from build123d import *

# Parameters (mm, degrees)
SKETCH2_W           = 90
SKETCH2_H           = 180
BOSS_EXTRUDE1_DEPTH = 10
BOSS_EXTRUDE2_START = 10
SKETCH2_3_R         = 5.5
SKETCH2_3_R_2       = 3.5
BOSS_EXTRUDE2_DEPTH = 5


with BuildPart() as part:
    # Sketch2 → Boss-Extrude1 (new body)
    with BuildSketch(Plane(origin=(0, 0, 0), x_dir=(1, 0, 0), z_dir=(0, 1, 0))):
        Rectangle(SKETCH2_W, SKETCH2_H)
    extrude(amount=BOSS_EXTRUDE1_DEPTH)

    # Sketch2<3> → Boss-Extrude2 (add)
    # profile 1 of 16: a face of its own
    with BuildSketch(Plane(origin=(0, 0, 0), x_dir=(1, 0, 0), z_dir=(0, 1, 0)).offset(BOSS_EXTRUDE2_START)):
        with Locations(Location((9.54, -80.46, 0), (0, 0, 90))):
            Circle(SKETCH2_3_R)
        with Locations(Location((9.54, -80.46, 0), (0, 0, 90))):
            Circle(SKETCH2_3_R_2, mode=Mode.SUBTRACT)
    # profile 2 of 16: a face of its own
    with BuildSketch(Plane(origin=(0, 0, 0), x_dir=(1, 0, 0), z_dir=(0, 1, 0)).offset(BOSS_EXTRUDE2_START)):
        with Locations(Location((35, -80.46, 0), (0, 0, 90))):
            Circle(SKETCH2_3_R)
        with Locations(Location((35, -80.46, 0), (0, 0, 90))):
            Circle(SKETCH2_3_R_2, mode=Mode.SUBTRACT)
    # profile 3 of 16: a face of its own
    with BuildSketch(Plane(origin=(0, 0, 0), x_dir=(1, 0, 0), z_dir=(0, 1, 0)).offset(BOSS_EXTRUDE2_START)):
        with Locations(Location((9.54, -55, 0), (0, 0, 90))):
            Circle(SKETCH2_3_R)
        with Locations(Location((9.54, -55, 0), (0, 0, 90))):
            Circle(SKETCH2_3_R_2, mode=Mode.SUBTRACT)
    # profile 4 of 16: a face of its own
    with BuildSketch(Plane(origin=(0, 0, 0), x_dir=(1, 0, 0), z_dir=(0, 1, 0)).offset(BOSS_EXTRUDE2_START)):
        with Locations(Location((35, -55, 0), (0, 0, 90))):
            Circle(SKETCH2_3_R)
        with Locations(Location((35, -55, 0), (0, 0, 90))):
            Circle(SKETCH2_3_R_2, mode=Mode.SUBTRACT)
    # profile 5 of 16: a face of its own
    with BuildSketch(Plane(origin=(0, 0, 0), x_dir=(1, 0, 0), z_dir=(0, 1, 0)).offset(BOSS_EXTRUDE2_START)):
        with Locations(Location((9.54, -35.46, 0), (0, 0, 90))):
            Circle(SKETCH2_3_R)
        with Locations(Location((9.54, -35.46, 0), (0, 0, 90))):
            Circle(SKETCH2_3_R_2, mode=Mode.SUBTRACT)
    # profile 6 of 16: a face of its own
    with BuildSketch(Plane(origin=(0, 0, 0), x_dir=(1, 0, 0), z_dir=(0, 1, 0)).offset(BOSS_EXTRUDE2_START)):
        with Locations(Location((35, -35.46, 0), (0, 0, 90))):
            Circle(SKETCH2_3_R)
        with Locations(Location((35, -35.46, 0), (0, 0, 90))):
            Circle(SKETCH2_3_R_2, mode=Mode.SUBTRACT)
    # profile 7 of 16: a face of its own
    with BuildSketch(Plane(origin=(0, 0, 0), x_dir=(1, 0, 0), z_dir=(0, 1, 0)).offset(BOSS_EXTRUDE2_START)):
        with Locations(Location((9.54, -10, 0), (0, 0, 90))):
            Circle(SKETCH2_3_R)
        with Locations(Location((9.54, -10, 0), (0, 0, 90))):
            Circle(SKETCH2_3_R_2, mode=Mode.SUBTRACT)
    # profile 8 of 16: a face of its own
    with BuildSketch(Plane(origin=(0, 0, 0), x_dir=(1, 0, 0), z_dir=(0, 1, 0)).offset(BOSS_EXTRUDE2_START)):
        with Locations(Location((35, -10, 0), (0, 0, 90))):
            Circle(SKETCH2_3_R)
        with Locations(Location((35, -10, 0), (0, 0, 90))):
            Circle(SKETCH2_3_R_2, mode=Mode.SUBTRACT)
    # profile 9 of 16: a face of its own
    with BuildSketch(Plane(origin=(0, 0, 0), x_dir=(1, 0, 0), z_dir=(0, 1, 0)).offset(BOSS_EXTRUDE2_START)):
        with Locations(Location((9.54, 9.54, 0), (0, 0, 90))):
            Circle(SKETCH2_3_R)
        with Locations(Location((9.54, 9.54, 0), (0, 0, 90))):
            Circle(SKETCH2_3_R_2, mode=Mode.SUBTRACT)
    # profile 10 of 16: a face of its own
    with BuildSketch(Plane(origin=(0, 0, 0), x_dir=(1, 0, 0), z_dir=(0, 1, 0)).offset(BOSS_EXTRUDE2_START)):
        with Locations(Location((35, 9.54, 0), (0, 0, 90))):
            Circle(SKETCH2_3_R)
        with Locations(Location((35, 9.54, 0), (0, 0, 90))):
            Circle(SKETCH2_3_R_2, mode=Mode.SUBTRACT)
    # profile 11 of 16: a face of its own
    with BuildSketch(Plane(origin=(0, 0, 0), x_dir=(1, 0, 0), z_dir=(0, 1, 0)).offset(BOSS_EXTRUDE2_START)):
        with Locations(Location((9.54, 35, 0), (0, 0, 90))):
            Circle(SKETCH2_3_R)
        with Locations(Location((9.54, 35, 0), (0, 0, 90))):
            Circle(SKETCH2_3_R_2, mode=Mode.SUBTRACT)
    # profile 12 of 16: a face of its own
    with BuildSketch(Plane(origin=(0, 0, 0), x_dir=(1, 0, 0), z_dir=(0, 1, 0)).offset(BOSS_EXTRUDE2_START)):
        with Locations(Location((35, 35, 0), (0, 0, 90))):
            Circle(SKETCH2_3_R)
        with Locations(Location((35, 35, 0), (0, 0, 90))):
            Circle(SKETCH2_3_R_2, mode=Mode.SUBTRACT)
    # profile 13 of 16: a face of its own
    with BuildSketch(Plane(origin=(0, 0, 0), x_dir=(1, 0, 0), z_dir=(0, 1, 0)).offset(BOSS_EXTRUDE2_START)):
        with Locations(Location((9.54, 54.54, 0), (0, 0, 90))):
            Circle(SKETCH2_3_R)
        with Locations(Location((9.54, 54.54, 0), (0, 0, 90))):
            Circle(SKETCH2_3_R_2, mode=Mode.SUBTRACT)
    # profile 14 of 16: a face of its own
    with BuildSketch(Plane(origin=(0, 0, 0), x_dir=(1, 0, 0), z_dir=(0, 1, 0)).offset(BOSS_EXTRUDE2_START)):
        with Locations(Location((35, 54.54, 0), (0, 0, 90))):
            Circle(SKETCH2_3_R)
        with Locations(Location((35, 54.54, 0), (0, 0, 90))):
            Circle(SKETCH2_3_R_2, mode=Mode.SUBTRACT)
    # profile 15 of 16: a face of its own
    with BuildSketch(Plane(origin=(0, 0, 0), x_dir=(1, 0, 0), z_dir=(0, 1, 0)).offset(BOSS_EXTRUDE2_START)):
        with Locations(Location((9.54, 80, 0), (0, 0, 90))):
            Circle(SKETCH2_3_R)
        with Locations(Location((9.54, 80, 0), (0, 0, 90))):
            Circle(SKETCH2_3_R_2, mode=Mode.SUBTRACT)
    # profile 16 of 16: a face of its own
    with BuildSketch(Plane(origin=(0, 0, 0), x_dir=(1, 0, 0), z_dir=(0, 1, 0)).offset(BOSS_EXTRUDE2_START)):
        with Locations(Location((35, 80, 0), (0, 0, 90))):
            Circle(SKETCH2_3_R)
        with Locations(Location((35, 80, 0), (0, 0, 90))):
            Circle(SKETCH2_3_R_2, mode=Mode.SUBTRACT)
    extrude(amount=BOSS_EXTRUDE2_DEPTH)


solid = part.part
Geometry: final body of the model. Coordinates: model frame, mm. A direction names the side the tool comes from. Give positions to 0.01 mm unless a question says otherwise; leave off trailing zeros. Write each loop counter-clockwise with the first axis right and the second up, starting at its lowest first coordinate (ties: lowest second). Pieces come first, ordered by that corner, then holes. Notation, with made-up numbers: (22, 32.25) - (66, 32.25) arc R21 cw to (66, 71.25) - close; hole circle Ø10 at (30, 6.25). An arc over 180 degrees is marked (long way). Return JSON: item names as keys, results as strings. Group by question number.
1) Section B-B on x = -28.5. Return the cut outline in (y, z), plus the area to 3 significant figures.
2) Set-up query: faces 4 (the cylindrical face through (7.175, 12.465, 12.58)), 5 (the flat face through (39, 15, -54)). Return all of +Z, -Z, +X, -X, +Y, -Y with unobstructed straight access to the full face (end or side cutting, diameter ignored); none if empty.
3) Line query: line 1 (X direction, y = 11.5, z = 10); line 2 (X direction, y = 13.25, z = 56); line 3 (Y direction, x = -28.5, z = -81). Output: solid intervals per line, ascending.
4) Section A-A on z = -35. Return the cut outline in (x, y).
5) Section C-C on z = -2. Return the cut outline in (x, y).
6) Mould query, pull axis Z, two halves, no side actions, for faces 1 (the flat face through (-1, 5, 90)), 2 (the flat face through (9, 15, 6)), 3 (the flat face through (35, 10, -10)). Classes: released by +Z, released by -Z, zero draft, split by the parting line, or undercut.
7) First-contact query: P1, Ø5, axis at x = -7.5, z = 37, coming from the +Y side; P2, Ø2, axis at x = 34, y = 12.5, coming from the +Z side. Flat tips, straight axial feed; report the tip coordinate or a pass-through.
Filled in:
{
 "1": {"outline": "(0, -90) - (10, -90) - (10, 90) - (0, 90) - close", "area": "1,800 mm^2"},
 "2": {"face 4": "+Y", "face 5": "+Z, -Z, +X, -X, +Y"},
 "3": {"line 1": "x = 4.04 to 6.04, 13.04 to 15.04, 29.5 to 31.5, 38.5 to 40.5", "line 2": "x = 4.13 to 6.19, 12.89 to 14.95, 29.59 to 31.65, 38.35 to 40.41", "line 3": "y = 0 to 10"},
 "4": {"outline": "(-45, 0) - (45, 0) - (45, 10) - (40.5, 10) - (40.5, 15) - (38.5, 15) - (38.5, 10) - (31.5, 10) - (31.5, 15) - (29.5, 15) - (29.5, 10) - (15.04, 10) - (15.04, 15) - (13.04, 15) - (13.04, 10) - (6.04, 10) - (6.04, 15) - (4.04, 15) - (4.04, 10) - (-45, 10) - close"},
 "5": {"outline": "(-45, 0) - (45, 0) - (45, 10) - (-45, 10) - close"},
 "6": {"face 1": "released by +Z", "face 2": "zero draft", "face 3": "undercut"},
 "7": {"P1": "stops at y = 10", "P2": "stops at z = 85.96"}
}
